Can you work these out from the drawing? Everything is in mm from the part's minimum corner. Give positions to 0.01 mm unless a question says otherwise; leave off trailing zeros. Write each loop counter-clockwise with the first axis right and the second up, starting at its lowest first coordinate (ties: lowest second). Pieces come first, ordered by that corner, then holes. Notation, with made-up numbers: (71, 43.25) - (100, 43.25) arc R24 ccw to (100, 66.25) - close; hole circle Ø6 at (82, 37.5). An arc over 180 degrees is marked (long way). Write each question's results on one line, items separated by ' | '. Start each with the question number.
Item 1: Suppose I cut it at B-B on z = 20.5. List the corners of the cut face in (x, y) for me.
Item 2: Will these pins go through, and if not, where does the flat tip stop? P1, Ø1.5, axis at y = 1.5, z = 2, coming from the -X side (1 decimal); P2, Ø1.5, axis at x = 49, y = 1, coming from the +Z side; P3, Ø0.9, axis at y = 1, z = 36, coming from the +X side.
Item 3: Suppose I cut it at A-A on x = 30. List the corners of the cut face in (y, z) for me.
Item 4: Please list where these lines run through material, in increasing order: line 1 along X through (y, z) = (1.1, 2) (1 decimal); line 2 along X through (y, z) = (2.45, 36.5); line 3 along Z through (x, y) = (39, 1.8).
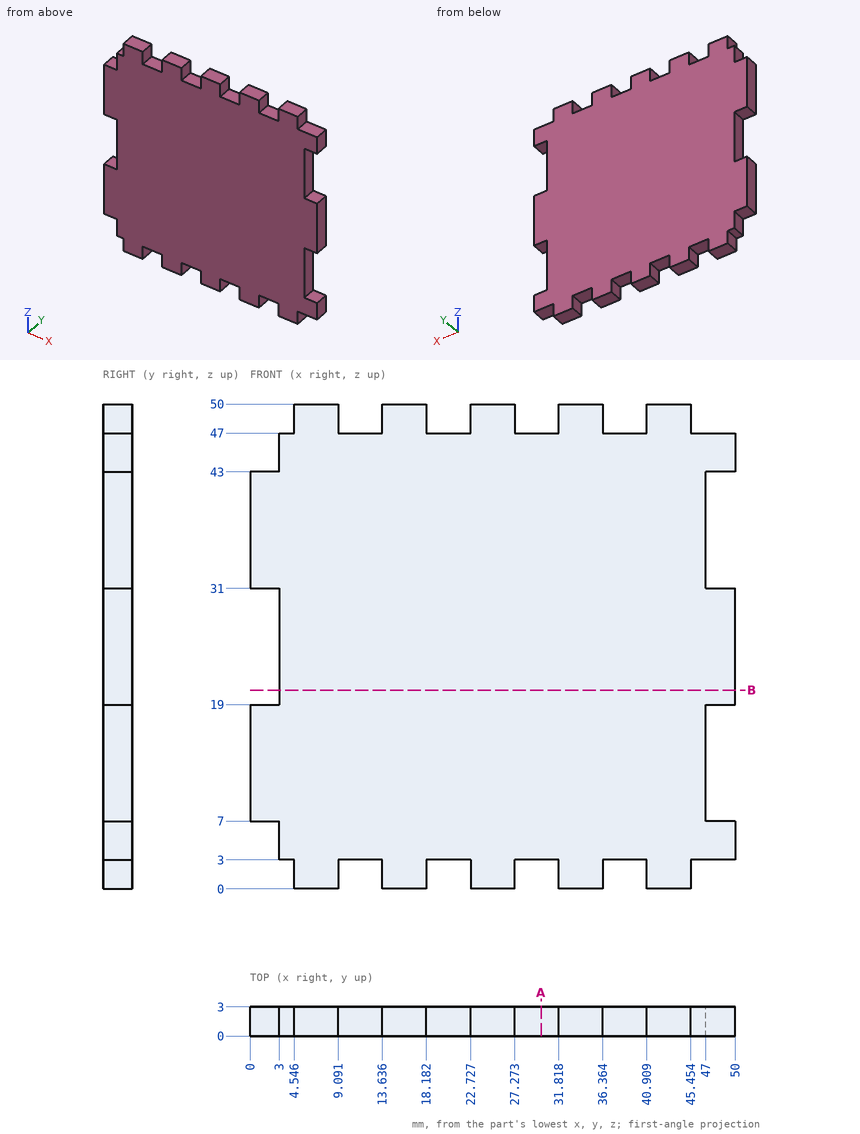
Checked values:
1) outline: (3, 0) - (50, 0) - (50, 3) - (3, 3) - close
2) P1: stops at x = 4.5 | P2: stops at z = 47 | P3: stops at x = 47
3) outline: (0, 3) - (3, 3) - (3, 47) - (0, 47) - close
4) line 1: x = 4.5 to 9.1, 13.6 to 18.2, 22.7 to 27.3, 31.8 to 36.4, 40.9 to 45.5 | line 2: x = 0 to 47 | line 3: z = 3 to 47
